Check sheet for the modelled part. Datum: model origin and axes. Units: mm. Face numbers are marked on the shaded views. A direction names the side the tool comes from. Give positions to 0.01 mm unless a question says otherwise; leave off trailing zeros. Loops run counter-clockwise (first coordinate to the right, second up) from the corner with the lowest first, then second, coordinate; pieces in that order, holes last. Notation, with made-up numbers: (83.25, 24.25) -> (93.25, 24.25) arc R20 ccw to (93.25, 53.25) -> close; hole circle Ø10 at (20, 75). An arc over 180 degrees is marked (long way). Answer as CSV lines item,"result". Start each with the question number.
(1) Section check C-C on x = 225.5. Enter the section's corners in (y, z), plus the area to 3 significant figures.
(2) Section check B-B on z = 91.5. Enter the section's corners in (x, y).
(3) Gauge pin test, flat ends, axial feed: pin 1 Ø3 at (y, z) = (6.5, 32.5) entering from +X; pin 2 Ø2 at (x, y) = (85, -7) entering from +Z; pin 3 Ø2 at (y, z) = (-5.5, 189) entering from -X. Record the tip position at first contact, or that the pin passes through.
(4) Material ranges on line 1 (X direction, y = 0, z = 81); line 2 (Z direction, x = 182, y = 1); line 3 (X direction, y = -1.5, z = 26.5), recorded low to high. Write a range as from..to.
(5) Section check D-D on z = 213.5. State how many separate pieces and enclosed holes the cut face has, plus the area to 3 significant figures.
(6) Access from +Z, -Z, +X, -X, +Y, -Y to the whole of each face (thin tool, end or side, straight path). Record for the marked faces 1 and 2.
(7) Section check A-A on y = 3.75. Enter the section's corners in (x, z), plus the area to 3 significant figures.
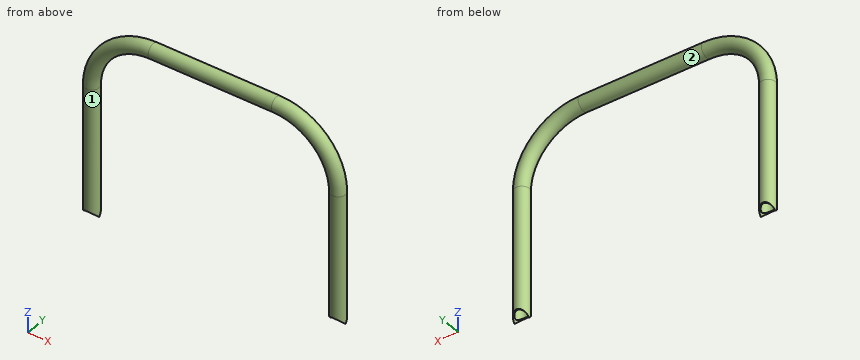
Solid Edge part; units mm, degrees
sketch "Sketch1" plane through (0, 0, 0) normal (0, -1, 0) x (1, 0, 0)
  line L0 (0, 0) -> (0, 170)
  arc A0 (0, 170) -> (80, 250) centre (80, 170) cw
  line L1 (80, 250) -> (240, 250)
  arc A1 (240, 250) -> (320, 170) centre (240, 170) cw
  line L2 (320, 170) -> (320, 0)
sketch "Sketch2" plane through (0, 0, 0) normal (0, 0, -1) x (-1, 0, 0)
  circle A0 centre (0, 0) radius 9.5
sweep "SweptProtrusion_1" add profiles "Sketch2" path "Sketch1"
shell "Thinwall_1" thickness 1.6 removed faces 4 at (6.5233, -6.1433, 0) at (313.4767, -6.1433, 0) at (6.5233, -6.1433, 0) at (313.4767, -6.1433, 0)
hole "Hole_3" at (0, 0, 0) direction (0, -1, 0) diameter 19 end through all both ways yes
hole "Hole1" at (320, 0, 0) direction (0, -1, 0) diameter 19 end through all both ways yes
properties material "Aluminum, 1060"
Working result:
1,outline,"circle Ø19 at (0, 250); hole circle Ø15.8 at (0, 250)"
1,area,"87.5 mm^2"
2,outline,"circle Ø19 at (0, 0); circle Ø19 at (320, 0); hole circle Ø15.8 at (0, 0); hole circle Ø15.8 at (320, 0)"
3,pin 1,"stops at x = 328.08"
3,pin 2,"stops at z = 257.37"
3,pin 3,"stops at x = -6.34"
4,line 1,"x = -9.5..-7.9, 7.9..9.5, 310.5..312.1, 327.9..329.5"
4,line 2,"z = 240.55..242.16, 257.84..259.45"
4,line 3,"x = -9.38..-7.76, 7.76..9.38, 310.62..312.24, 327.76..329.38"
5,separate pieces,"2"
5,enclosed holes,"2"
5,area,"210 mm^2"
6,face 1,"-Z"
6,face 2,"none"
7,outline,"(-8.73, 3.75) arc R9.5 cw to (-6.95, 6.47) -> (-6.95, 170) arc R86.95 cw to (80, 256.95) -> (240, 256.95) arc R86.95 cw to (326.95, 170) -> (326.95, 6.47) arc R9.5 cw to (328.73, 3.75) -> (328.73, 170) arc R88.73 ccw to (240, 258.73) -> (80, 258.73) arc R88.73 ccw to (-8.73, 170) -> close; (6.95, 6.47) arc R9.5 cw to (8.73, 3.75) -> (8.73, 170) arc R71.27 cw to (80, 241.27) -> (240, 241.27) arc R71.27 cw to (311.27, 170) -> (311.27, 3.75) arc R9.5 cw to (313.05, 6.47) -> (313.05, 170) arc R73.05 ccw to (240, 243.05) -> (80, 243.05) arc R73.05 ccw to (6.95, 170) -> close"
7,area,"2,630 mm^2"
